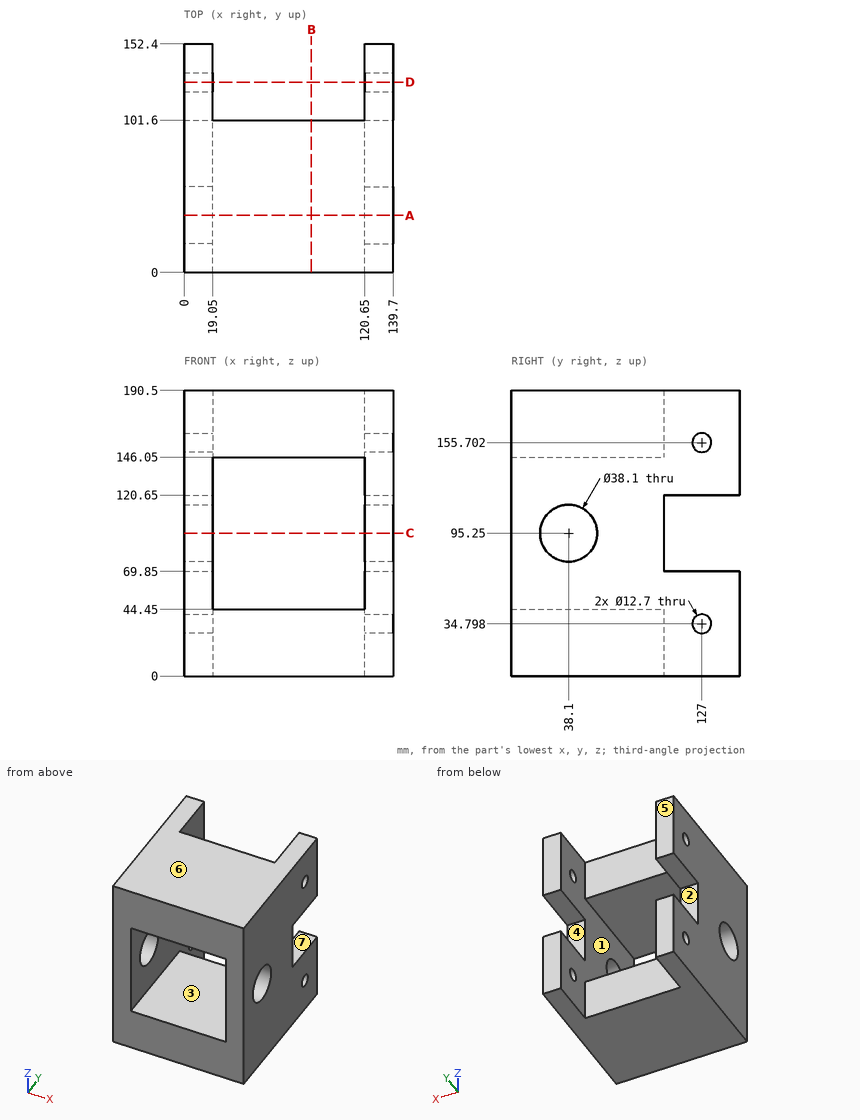
Source: three-view drawing plus pictorial views. Frame: mm from the lowest corner of the part. A direction names the side the tool comes from. Round coordinates to 2 decimals unless told otherwise and drop trailing zeros. Loops run counter-clockwise (first coordinate to the right, second up) from the corner with the lowest first, then second, coordinate; pieces in that order, holes last.
1. Access query for the marked faces 1, 2 and 3. Directions: +Z, -Z, +X, -X, +Y, -Y. A direction counts if a zero-diameter tool reaches every point of the face in a straight line with its end or side. Return the directions, or none.
2. Section query A-A on y = 38.1. Output: boundary loops of the cut face in (x, z).
3. Section query C-C on z = 95.25. Output: boundary loops of the cut face in (x, y).
4. Contact query for flat-ended pins moving along their axis: pin 1 (5.5 mm diameter, centred on x = 5, z = 94.5, fed in from +Y); pin 2 (23 mm diameter, centred on y = 38.1, z = 95.25, fed in from +X). Output: stop coordinate, or through.
5. Section query B-B on x = 85. Output: boundary loops of the cut face in (y, z).
6. Mould query, pull axis Z, two halves, no side actions, for the marked faces 4, 5, 6 and 7. Classes: released by +Z, released by -Z, zero draft, split by the parting line, or undercut.
7. Section query D-D on y = 127. Give the number of separate pieces and of enclosed holes in the cut face, and give its area (3 significant figures).
8. Ray query, L1, parallel to Z at x = 93, y = 75; L2, parallel to X at y = 141.5, z = 48; L3, parallel to Y at x = 14, z = 95. Return the intervals inside material, ascending.
Answers below:
1. face 1: +Y
1. face 2: +X, -X, +Y
1. face 3: +Y, -Y
2. outline: (0, 0) - (139.7, 0) - (139.7, 76.2) - (120.65, 76.2) - (120.65, 44.45) - (19.05, 44.45) - (19.05, 76.2) - (0, 76.2) - close; (0, 114.3) - (19.05, 114.3) - (19.05, 146.05) - (120.65, 146.05) - (120.65, 114.3) - (139.7, 114.3) - (139.7, 190.5) - (0, 190.5) - close
3. outline: (0, 0) - (19.05, 0) - (19.05, 19.05) - (0, 19.05) - close; (0, 57.15) - (19.05, 57.15) - (19.05, 101.6) - (0, 101.6) - close; (120.65, 0) - (139.7, 0) - (139.7, 19.05) - (120.65, 19.05) - close; (120.65, 57.15) - (139.7, 57.15) - (139.7, 101.6) - (120.65, 101.6) - close
4. pin 1: stops at y = 101.6
4. pin 2: passes through
5. outline: (0, 0) - (101.6, 0) - (101.6, 44.45) - (0, 44.45) - close; (0, 146.05) - (101.6, 146.05) - (101.6, 190.5) - (0, 190.5) - close
6. face 4: undercut
6. face 5: zero draft
6. face 6: released by +Z
6. face 7: undercut
7. separate pieces: 8
7. enclosed holes: 0
7. area: 4,350 mm2
8. L1: z = 0 to 44.45, 146.05 to 190.5
8. L2: x = 0 to 19.05, 120.65 to 139.7
8. L3: y = 0 to 19.05, 57.15 to 101.6
